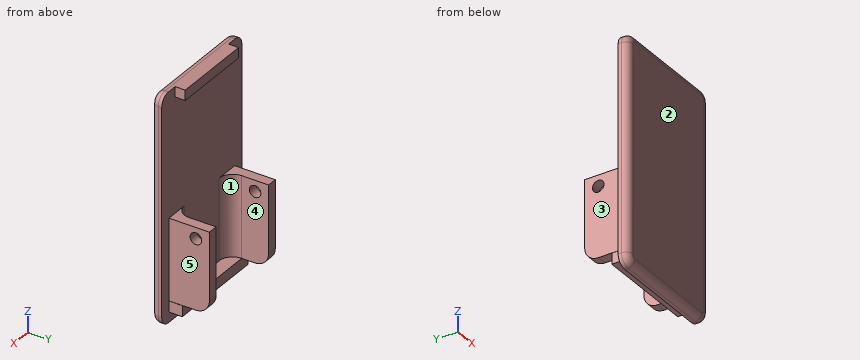
```python
from build123d import *

# Parameters (mm, degrees)
SKETCH_1_W          = 18
SKETCH_1_H          = 33.5
EXTRUDE_1_DEPTH     = 1.5
FILLET_1_R          = 1.5
SKETCH_2_W          = 1.5
SKETCH_2_H          = 12
EXTRUDE_2_DEPTH     = 6
SKETCH_3_W          = 14.8
SKETCH_3_H          = 1.6
EXTRUDE_3_DEPTH     = 2
FILLET_2_R          = 2
SKETCH_4_R          = 0.856485036
CUT_EXTRUDE_1_DEPTH = 18
SKETCH_5_W          = 12
SKETCH_5_H          = 1.5
EXTRUDE_4_DEPTH     = 1.5
FILLET_3_R          = 1


with BuildPart() as part:
    # 草图1 → 凸台-拉伸1 (new body)
    with BuildSketch(Plane(origin=(0, 0, 0), x_dir=(1, 0, 0), z_dir=(0, 1, 0))):
        Rectangle(SKETCH_1_W, SKETCH_1_H)
    extrude(amount=EXTRUDE_1_DEPTH)

    # 圆角1
    fillet_1_edges = [part.edges().sort_by_distance(p)[0] for p in [
        (-9, 0.75, -16.75),
        (9, 0.75, -16.75),
        (9, 0.75, 16.75),
        (-9, 0.75, 16.75),
    ]]
    fillet(fillet_1_edges, radius=FILLET_1_R)

    # 草图2 → 凸台-拉伸2 (add)
    with BuildSketch(Plane(origin=(0, 1.5, 0), x_dir=(1, 0, 0), z_dir=(0, 1, 0))):
        with Locations((-6.65, 7.622409508)):
            Rectangle(SKETCH_2_W, SKETCH_2_H)
        with Locations((6.65, 7.622409508)):
            Rectangle(SKETCH_2_W, SKETCH_2_H)
    extrude(amount=EXTRUDE_2_DEPTH)

    # 草图3 → 凸台-拉伸3 (add)
    with BuildSketch(Plane(origin=(0, 1.5, 0), x_dir=(1, 0, 0), z_dir=(0, 1, 0))):
        with Locations((0, 14.45)):
            Rectangle(SKETCH_3_W, SKETCH_3_H)
    extrude(amount=EXTRUDE_3_DEPTH)

    # 圆角2
    fillet_2_edges = [part.edges().sort_by_distance(p)[0] for p in [
        (-5.9, 1.5, -7.622409508),
        (-6.65, 7.5, -13.622409508),
        (5.9, 1.5, -7.622409508),
        (6.65, 7.5, -13.622409508),
    ]]
    fillet(fillet_2_edges, radius=FILLET_2_R)

    # 草图4 → 切除-拉伸1 (cut)
    with BuildSketch(Plane(origin=(7.4, 0, 0), x_dir=(0, 0, -1), z_dir=(1, 0, 0))):
        with Locations((3.25, 5.5)):
            Circle(SKETCH_4_R)
    extrude(amount=-CUT_EXTRUDE_1_DEPTH, mode=Mode.SUBTRACT)

    # 草图5 → 凸台-拉伸4 (add)
    with BuildSketch(Plane(origin=(0, 1.5, 0), x_dir=(1, 0, 0), z_dir=(0, 1, 0))):
        with Locations((0, -16)):
            Rectangle(SKETCH_5_W, SKETCH_5_H)
    extrude(amount=EXTRUDE_4_DEPTH)

    # 圆角3
    fillet_3_edges = [part.edges().sort_by_distance(p)[0] for p in [
        (9, 0, 0),
        (-9, 0, 0),
        (0, 0, -16.75),
        (0, 0, 16.75),
        (-8.560660172, 0, -16.310660172),
        (8.560660172, 0, -16.310660172),
        (-8.560660172, 0, 16.310660172),
        (8.560660172, 0, 16.310660172),
    ]]
    fillet(fillet_3_edges, radius=FILLET_3_R)


solid = part.part
```
The listing builds one solid part. Answer for the finished solid, in the listing's coordinates (mm). Face numbers are marked on the shaded views. A direction names the side the tool comes from. Coordinates: 2 decimals unless noted, no trailing zeros. Write each loop counter-clockwise with the first axis right and the second up, starting at its lowest first coordinate (ties: lowest second). Pieces come first, ordered by that corner, then holes.
Q1. Which of the six approach directions +Z, -Z, +X, -X, +Y, -Y give full straight-line access (tool end or side, diameter ignored) to the marked faces 3, 4 and 5?
Returned:
face 3: +Z, -Z, -X, +Y
face 4: +Z, -Z, +Y
face 5: +Z, -Z, +X, +Y
Q2. Section C-C, the plane y = 2.25 is taken. Write down the section's boundary in (x, z).
Returned:
outline: (-7.4, -15.25) - (7.4, -15.25) - (7.4, -13.65) - (-7.4, -13.65) - close; (-7.4, -13.62) - (-5.46, -13.62) - (-5.46, -1.62) - (-7.4, -1.62) - close; (-6, 15.25) - (6, 15.25) - (6, 16.75) - (-6, 16.75) - close; (5.46, -13.62) - (7.4, -13.62) - (7.4, -1.62) - (5.46, -1.62) - close
Q3. Find the intervals of material crossed by line 1 along Y through (x, z) = (-6.25, -3.25); line 2 along X through (y, z) = (7, -9.5); line 3 along Y through (x, z) = (6.75, -14.5), in increasing order.
Returned:
line 1: y = 0 to 4.64, 6.36 to 7.5
line 2: x = -7.4 to -5.9, 5.9 to 7.4
line 3: y = 0 to 3.5
Q4. Section A-A, the plane z = -4.5 is taken. Write down the section's boundary in (x, y).
Returned:
outline: (-9, 1) arc R1 ccw to (-8, 0) - (8, 0) arc R1 ccw to (9, 1) - (9, 1.5) - (7.4, 1.5) - (7.4, 7.5) - (5.9, 7.5) - (5.9, 3.5) arc R2 cw to (3.9, 1.5) - (-3.9, 1.5) arc R2 cw to (-5.9, 3.5) - (-5.9, 7.5) - (-7.4, 7.5) - (-7.4, 1.5) - (-9, 1.5) - close
Q5. Section B-B, the plane x = -1.75 is taken. Write down the section's boundary in (y, z), then the cut area to 3 significant figures.
Returned:
outline: (0, -15.75) arc R1 ccw to (1, -16.75) - (1.5, -16.75) - (1.5, -15.25) - (3.5, -15.25) - (3.5, -13.65) - (1.5, -13.65) - (1.5, 15.25) - (3, 15.25) - (3, 16.75) - (1, 16.75) arc R1 ccw to (0, 15.75) - close
area: 55.3 mm2
Q6. Given P1, Ø1, axis at x = 5, y = 2.5, coming from the -Z side; P2, Ø4, axis at x = 5.5, y = 5.5, coming from the +Z side; P3, Ø0.8, axis at x = 0, z = 16, coming from the +Y side; P4, Ø1, axis at y = 3, z = 9.5, coming from the -X side, each flat-ended and moving along its own axis, determine where each tip first touches the part or whether it passes through.
Returned:
P1: stops at z = -15.25
P2: stops at z = -1.62
P3: stops at y = 3
P4: passes through
Q7. The mould has two halves that part along Z. Classify the marked faces 1 and 2: released by +Z, released by -Z, zero draft, split by the parting line, or undercut.
Returned:
face 1: undercut
face 2: zero draft
Q8. Section D-D, the plane z = 10 is taken. Write down the section's boundary in (x, y).
Returned:
outline: (-9, 1) arc R1 ccw to (-8, 0) - (8, 0) arc R1 ccw to (9, 1) - (9, 1.5) - (-9, 1.5) - close
